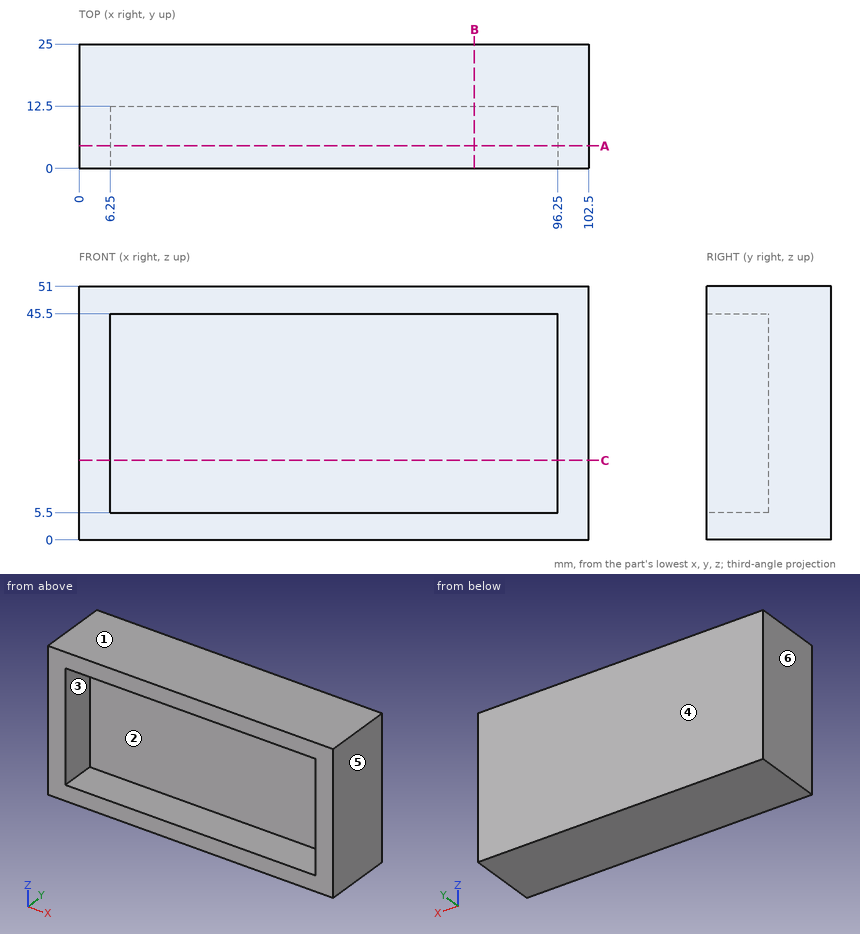
Print and shaded views of the part. All mm, measured from the part's lowest x, y and z. A direction names the side the tool comes from. Give positions to 0.01 mm unless a question says otherwise; leave off trailing zeros. Loops run counter-clockwise (first coordinate to the right, second up) from the corner with the lowest first, then second, coordinate; pieces in that order, holes last. Notation, with made-up numbers: (-0.5, 13) -> (15.5, 13) arc R28 ccw to (15.5, 42) -> close; hole circle Ø9 at (10.5, 71). An arc over 180 degrees is marked (long way). One line per question, with ' | ' between items. Start each with the question number.
1) Pin check, flat tips, straight feed: pin 1 (10 mm diameter, centred on x = 64.5, y = 7.5, fed in from -Z); pin 2 (10 mm diameter, centred on x = 30, z = 20, fed in from -Y). Stop position of each tip, or through.
2) Two-plate mould, pull along X, no slides. Class the marked faces 3, 4, 5 and 6: released by +X, released by -X, zero draft, split by the parting line, or undercut.
3) Cut at A-A (y = 4.5). Give the cut face in (x, z), plus the area to 3 significant figures.
4) 3-axis set-ups, long thin cutter, end or side, ignore diameter. For the marked faces 1 and 2: which of +Z, -Z, +X, -X, +Y, -Y reach the whole face in a straight line?
5) Cut at B-B (x = 79.5). Give the cut face in (y, z), plus the area to 3 significant figures.
6) Cut at C-C (z = 16). Give the cut face in (x, y).
7) Probe L1, parallel to X at y = 9, z = 43; L2, parallel to Z at x = 75, y = 7; L3, parallel to Y at x = 80.5, z = 7. List the from-to ranges inside material, lowest first.
Return value:
1) pin 1: z = 0 | pin 2: y = 12.5
2) face 3: undercut | face 4: zero draft | face 5: released by +X | face 6: released by -X
3) outline: (0, 0) -> (102.5, 0) -> (102.5, 51) -> (0, 51) -> close; hole (6.25, 5.5) -> (96.25, 5.5) -> (96.25, 45.5) -> (6.25, 45.5) -> close | area: 1,630 mm^2
4) face 1: +Z, +X, -X, +Y, -Y | face 2: -Y
5) outline: (0, 0) -> (25, 0) -> (25, 51) -> (0, 51) -> (0, 45.5) -> (12.5, 45.5) -> (12.5, 5.5) -> (0, 5.5) -> close | area: 775 mm^2
6) outline: (0, 0) -> (6.25, 0) -> (6.25, 12.5) -> (96.25, 12.5) -> (96.25, 0) -> (102.5, 0) -> (102.5, 25) -> (0, 25) -> close
7) L1: 0 to 6.25, 96.25 to 102.5 | L2: 0 to 5.5, 45.5 to 51 | L3: 12.5 to 25
